from build123d import *

# Parameters (mm, degrees)
F1_DEPTH = 4
F2_R     = 5
F3_T     = -1.5
F4_R     = 1.5
F5_DEPTH = 3
F6_R     = 0.75
F7_DEPTH = 1.5


with BuildPart() as f1:
    # F0 (on Top) → F1 (new body)
    with BuildSketch(Plane.XY):
        with BuildLine():
            ThreePointArc((-7.794229, 4.5), (-5.011221, 7.475805), (-1.201188, 8.919481))
            Line((-1.201188, 8.919481), (9.473696, 27.408923))
            ThreePointArc((9.473696, 27.408923), (29, 0), (9.473696, -27.408923))
            Line((9.473696, -27.408923), (-1.201188, -8.919481))
            ThreePointArc((-1.201188, -8.919481), (-5.011221, -7.475805), (-7.794229, -4.5))
            Line((-7.794229, -4.5), (7.820268, -31.545101))
            ThreePointArc((7.820268, -31.545101), (32.5, 0), (7.820268, 31.545101))
            Line((7.820268, 31.545101), (-7.794229, 4.5))
        make_face()
        with BuildLine():
            ThreePointArc((-1.201188, -8.919481), (5.924074, -6.775348), (9, 0))
            ThreePointArc((9, 0), (5.924074, 6.775348), (-1.201188, 8.919481))
            ThreePointArc((-1.201188, 8.919481), (-5.011221, 7.475805), (-7.794229, 4.5))
            ThreePointArc((-7.794229, 4.5), (-9, 0), (-7.794229, -4.5))
            ThreePointArc((-7.794229, -4.5), (-5.011221, -7.475805), (-1.201188, -8.919481))
        make_face()
    extrude(amount=F1_DEPTH)

    # F2
    f2_edges = [f1.edges().sort_by_distance(p)[0] for p in [
        (9.473696, 27.408923, 2),
        (9.473696, -27.408923, 2),
        (7.820268, 31.545101, 2),
        (-1.201188, -8.919481, 2),
        (-1.201188, 8.919481, 2),
        (7.820268, -31.545101, 2),
    ]]
    fillet(f2_edges, radius=F2_R)

    # F3
    f3_openings = [f1.faces().sort_by_distance(p)[0] for p in [
        (7.079481, -4.25771, 4),
    ]]
    offset(amount=F3_T, openings=f3_openings)

    # F4 (on Top) → F5 (cut)
    with BuildSketch(Plane.XY):
        Circle(F4_R)
    extrude(amount=F5_DEPTH, mode=Mode.SUBTRACT)

    # F6 (on Top) → F7 (cut, through all)
    with BuildSketch(Plane.XY):
        with Locations((2.934493, 2.934493)):
            Circle(F6_R)
        with Locations((-2.934493, 2.934493)):
            Circle(F6_R)
        with Locations((-2.934493, -2.934493)):
            Circle(F6_R)
        with Locations((2.934493, -2.934493)):
            Circle(F6_R)
    extrude(amount=F7_DEPTH, mode=Mode.SUBTRACT)


solid = f1.part
Check sheet for the modelled part. Datum: model origin and axes. Units: mm. A direction names the side the tool comes from. Round coordinates to 2 decimals unless told otherwise and drop trailing zeros. Order: outer loops, then holes, each group sorted by start corner. A loop starts at its lowest first (then second) coordinate and runs counter-clockwise, first axis right, second up. Notation, with made-up numbers: M 54,88 L 86,88 A13 ccw 86,93 Z; hole C 77.25,31.5 d10. An arc over 180 degrees is marked long. One line per item, written item: value. Start each with the question number.
1. Access from +Z, -Z, +X, -X, +Y, -Y to the whole of each face (thin tool, end or side, straight path). Record for faces 1 (the cylindrical face through (10.27, -25.86, 2.03)), 2 (the flat face through (3, 0, 1.5)), 3 (the flat face through (-1.088, -16.116, 1.972)).
2. Gauge pin test, flat ends, axial feed: P1, Ø2, axis at x = 2.93, y = 2.93, coming from the -Z side; P2, Ø3.5, axis at x = 0, y = 0, coming from the +Z side; P3, Ø0.9, axis at x = -2.93, y = 2.93, coming from the +Z side; P4, Ø1.5, axis at x = -3, z = 1, coming from the -Y side. Record the tip position at first contact, or that the pin passes through.
3. Section check A-A on z = 2.85. Give the number of separate pieces and of enclosed holes in the cut face, and give its area (3 significant figures).
4. Section check C-C on x = 20. Enter the section's corners in (y, z).
5. Release check for a two-part mould opening along Y. For faces 4 (the flat face through (-0.897, 16.446, 1.972)), 5 (the flat face through (8, 0, 4)), 6 (the cylindrical face through (10.17, 25.83, 2.03)), 7 (the cylindrical face through (9.88, -27.31, 2.77)) record: released by +Y, released by -Y, zero draft, split by the parting line, or undercut.
6. Scan lines: line 1 along Y through (x, z) = (4.5, 0.7); line 2 along X through (y, z) = (6, 1.55); line 3 along Y through (x, z) = (2, 1.6). Record each from-to range of solid material in increasing order.
7. Section check B-B on y = -21. Enter the section's corners in (x, z).
Results found:
1. face 1: +Z, -Z
1. face 2: +Z
1. face 3: +Z, -Z, -X, -Y
2. P1: z = 0
2. P2: z = 1.5
2. P3: through
2. P4: y = -14.1
3. separate pieces: 2
3. enclosed holes: 2
3. area: 433 mm^2
4. outline: M -25.62,0 L -21,0 L -21,4 L -23.03,4 L -23.03,1.5 L -23.69,1.5 L -23.69,4 L -25.62,4 Z; M 21,0 L 25.62,0 L 25.62,4 L 23.69,4 L 23.69,1.5 L 23.03,1.5 L 23.03,4 L 21,4 Z
5. face 4: released by +Y
5. face 5: zero draft
5. face 6: undercut
5. face 7: undercut
6. line 1: -25.79 to -18.79, -7.79 to 7.79, 18.79 to 25.79
6. line 2: -6.93 to -5.2, 4.5 to 6.71, 28.37 to 29.9, 30.41 to 31.94
6. line 3: -21.46 to -18.46, -17.46 to -14.41, -10.32 to -7.74, 7.74 to 10.32, 14.41 to 17.46, 18.46 to 21.46
7. outline: M 1.73,0 L 5.77,0 L 5.77,4 L 4.04,4 L 4.04,1.5 L 3.46,1.5 L 3.46,4 L 1.73,4 Z; M 20,0 L 24.8,0 L 24.8,4 L 22.8,4 L 22.8,1.5 L 22.12,1.5 L 22.12,4 L 20,4 Z
